Geometry: see drawing. Coordinates: mm, zero at the bounding-box minimum. Coordinates: 2 decimals unless noted, no trailing zeros. Order: outer loops, then holes, each group sorted by start corner. A loop starts at its lowest first (then second) coordinate and runs counter-clockwise, first axis right, second up. Notation, with made-up numbers: M 79,30.5 L 112,30.5 A13 cw 112,49.5 Z; hole C -6,8 d2. An arc over 180 degrees is marked long. Answer in a Markdown table with one row per item.
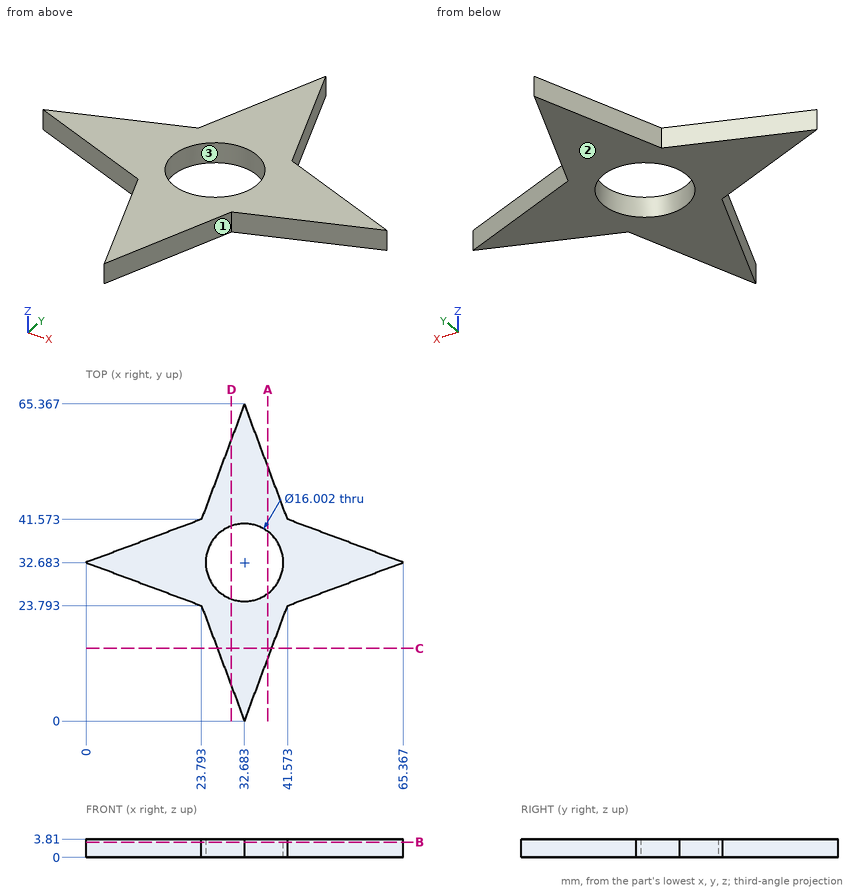
1) Mould query, pull axis X, two halves, no side actions, for the marked faces 1, 2 and 3. Classes: +X half, -X half, draft (parallel to the pull), parting line (faces both ways), or undercut.
Resolved:
| item | result |
|---|---|
| face 1 | +X half |
| face 2 | draft |
| face 3 | undercut |
2) Contact query for flat-ended pins moving along their axis: pin 1 (1.5 mm diameter, centred on x = 13, z = 2.5, fed in from +Y); pin 2 (1 mm diameter, centred on x = 23, z = 0.5, fed in from -Y). Output: stop coordinate, or through.
Resolved:
| item | result |
|---|---|
| pin 1 | stops at y = 37.82 |
| pin 2 | stops at y = 23.9 |
3) Cut plane B-B, the plane z = 3.15. Output: boundary loops of the cut face in (x, y) (1 decimal), and give its area (3 significant figures).
Resolved:
| item | result |
|---|---|
| outline | M 0,32.7 L 23.8,23.8 L 32.7,0 L 41.6,23.8 L 65.4,32.7 L 41.6,41.6 L 32.7,65.4 L 23.8,41.6 Z; hole C 32.7,32.7 d16 |
| area | 961 mm2 |
4) Cut plane D-D, the plane x = 30. Output: boundary loops of the cut face in (y, z) (1 decimal).
Resolved:
| item | result |
|---|---|
| outline | M 7.2,0 L 25.1,0 L 25.1,3.8 L 7.2,3.8 Z; M 40.2,0 L 58.2,0 L 58.2,3.8 L 40.2,3.8 Z |
5) Cut plane A-A, the plane x = 37.5. Output: boundary loops of the cut face in (y, z) (1 decimal), and give its area (3 significant figures).
Resolved:
| item | result |
|---|---|
| outline | M 12.9,0 L 26.3,0 L 26.3,3.8 L 12.9,3.8 Z; M 39.1,0 L 52.5,0 L 52.5,3.8 L 39.1,3.8 Z |
| area | 102 mm2 |
6) Cut plane C-C, the plane y = 15. Output: boundary loops of the cut face in (x, z), and give its area (3 significant figures).
Resolved:
| item | result |
|---|---|
| outline | M 27.08,0 L 38.29,0 L 38.29,3.81 L 27.08,3.81 Z |
| area | 42.7 mm2 |
7) Material intervals for probe 1 along Y at (x, z) = (7.5, 0.75) (1 decimal); probe 2 along X at (y, z) = (42, 2.95) (1 decimal); probe 3 along Y at (x, z) = (19.5, 0.9), sorted ascending.
Resolved:
| item | result |
|---|---|
| probe 1 | y = 29.9 to 35.5 |
| probe 2 | x = 24 to 41.4 |
| probe 3 | y = 25.4 to 39.97 |
